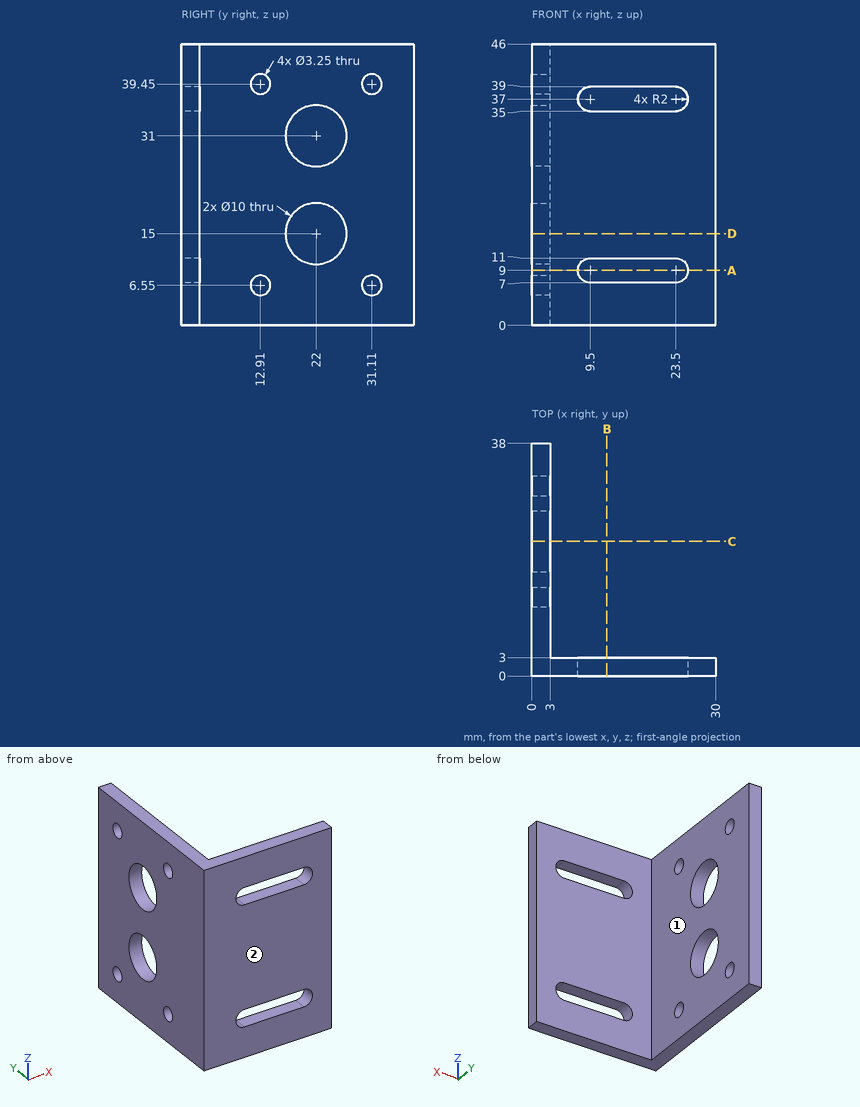
Job drawing, mm, ordinate dimensions from the low corner. One solid piece. A direction names the side the tool comes from. Coordinates: 2 decimals unless noted, no trailing zeros. Order: outer loops, then holes, each group sorted by start corner. A loop starts at its lowest first (then second) coordinate and runs counter-clockwise, first axis right, second up. Notation, with made-up numbers: (89.25, 37.5) - (97.25, 37.5) arc R27 cw to (97.25, 74.5) - close; hole circle Ø2 at (-23, 12.5). An arc over 180 degrees is marked (long way). Return JSON: item names as keys, results as strings. Group by question number.
1) Probe line 1 (Y direction, x = 2.1, z = 39.45) (3 decimals); line 2 (Z direction, x = 10.25, y = 2); line 3 (X direction, y = 6.5, z = 34). List the from-to ranges inside material, lowest first. Write a range as from..to.
2) Saw through at D-D, the plane z = 15. Write the cut outline in (x, y).
3) Saw through at B-B, the plane x = 12.25. Write the cut outline in (y, z).
4) Saw through at A-A, the plane z = 9. Write the cut outline in (x, y).
5) Flat gauge pins, fed straight in: P1, Ø1.5, axis at y = 25, z = 22, coming from the +X side; P2, Ø6, axis at y = 22, z = 31, coming from the -X side. Where does each tip first touch, or does it go through?
6) Tool access for the marked faces 1 and 2: list every direction of +Z, -Z, +X, -X, +Y, -Y with a clear straight run to the whole face (end or side of a thin tool).
7) Saw through at C-C, the plane y = 22. Write the cut outline in (x, z).
Values found:
{
 "1": {"line 1": "y = 0..11.285, 14.535..29.485, 32.735..38", "line 2": "z = 0..7, 11..35, 39..46", "line 3": "x = 0..3"},
 "2": {"outline": "(0, 0) - (30, 0) - (30, 3) - (3, 3) - (3, 17) - (0, 17) - close; (0, 27) - (3, 27) - (3, 38) - (0, 38) - close"},
 "3": {"outline": "(0, 0) - (3, 0) - (3, 7) - (0, 7) - close; (0, 11) - (3, 11) - (3, 35) - (0, 35) - close; (0, 39) - (3, 39) - (3, 46) - (0, 46) - close"},
 "4": {"outline": "(0, 0) - (7.5, 0) - (7.5, 3) - (3, 3) - (3, 38) - (0, 38) - close; (25.5, 0) - (30, 0) - (30, 3) - (25.5, 3) - close"},
 "5": {"P1": "stops at x = 3", "P2": "passes through"},
 "6": {"face 1": "+Z, -Z, +X, +Y", "face 2": "+Z, -Z, +X, -X, -Y"},
 "7": {"outline": "(0, 0) - (3, 0) - (3, 10) - (0, 10) - close; (0, 20) - (3, 20) - (3, 26) - (0, 26) - close; (0, 36) - (3, 36) - (3, 46) - (0, 46) - close"}
}
